The model under review builds one solid part; all positions refer to its coordinate system, in mm. Face numbers are marked on the shaded views. A direction names the side the tool comes from. Round coordinates to 2 decimals unless told otherwise and drop trailing zeros. Write each loop counter-clockwise with the first axis right and the second up, starting at its lowest first coordinate (ties: lowest second). Pieces come first, ordered by that corner, then holes. Notation, with made-up numbers: (64, -36.5) -> (122, -36.5) arc R28 cw to (122, -6.5) -> close; hole circle Ø11 at (30.5, 1). An arc over 180 degrees is marked (long way). Use CSV: the item, a comma, the result in double quotes. Start each with the question number.
1) Machinability: for the marked faces 1 and 2, which of the approach directions +Z, -Z, +X, -X, +Y, -Y give a long, thin tool a straight path to every point of the face, cutting with its end or side? Answer none if there is none.
2) Wall thickness on probe 1 along Y at (x, z) = (0, 1.2); probe 2 along X at (y, z) = (3, 4); probe 3 along Y at (x, z) = (1, 3.6): over which ranges is each line inside the solid? List them lowest first. Write a range as [from, to].
3) Take a section at A-A, the plane y = 0. State how many separate pieces and enclosed holes the cut face has, then the cut area to 3 significant figures.
4) Mouldability with a two-part tool opening along X and no side actions: class the marked faces 3 and 4 as released by +X, released by -X, zero draft, split by the parting line, or undercut.
5) For pin 1 Ø8.5 at (x, y) = (-29, 0) entering from +Z; pin 2 Ø18.5 at (x, y) = (-7, -2) entering from -Z; pin 3 Ø1 at (y, z) = (-20, 1) entering from +X, all flat-tipped, find the tip position at first contact; note any pin that passes through.
6) Take a section at B-B, the plane z = 3.3. Give the boundary of the cut face in (x, y).
from build123d import *

# Parameters (mm, degrees)
F0_R     = 37
F0_R_2   = 3.25
F1_DEPTH = 5
F2_SIZE  = 2.75
F3_SIZE  = 0.5
F4_R     = 19
F5_DEPTH = 2
F6_SIZE  = 0.5


with BuildPart() as f1:
    # F0 (on Top) → F1 (new body)
    with BuildSketch(Plane.XY):
        Circle(F0_R)
        with Locations((0, -29)):
            Circle(F0_R_2, mode=Mode.SUBTRACT)
        with Locations((-29, 0)):
            Circle(F0_R_2, mode=Mode.SUBTRACT)
        with Locations((29, 0)):
            Circle(F0_R_2, mode=Mode.SUBTRACT)
        with Locations((0, 29)):
            Circle(F0_R_2, mode=Mode.SUBTRACT)
    extrude(amount=F1_DEPTH)

    # F2
    f2_edges = [f1.edges().sort_by_distance(p)[0] for p in [
        (-3.25, -29, 5),
        (-32.25, 0, 5),
        (-3.25, 29, 5),
        (25.75, 0, 5),
    ]]
    chamfer(f2_edges, length=F2_SIZE)

    # F3
    f3_edges = [f1.edges().sort_by_distance(p)[0] for p in [
        (37, 0, 2.5),
        (-37, 0, 0),
        (-37, 0, 5),
        (-3.25, -29, 0),
        (-32.25, 0, 0),
        (-3.25, 29, 0),
        (25.75, 0, 0),
    ]]
    chamfer(f3_edges, length=F3_SIZE)

    # F4 (on face) → F5 (cut)
    with BuildSketch(Plane(origin=(0, 0, 0), x_dir=(1, 0, 0), z_dir=(0, 0, -1))):
        Circle(F4_R)
    extrude(amount=-F5_DEPTH, mode=Mode.SUBTRACT)

    # F6
    f6_edges = [f1.edges().sort_by_distance(p)[0] for p in [
        (19, 0, 1),
        (-19, 0, 0),
        (-19, 0, 2),
    ]]
    chamfer(f6_edges, length=F6_SIZE)


solid = f1.part
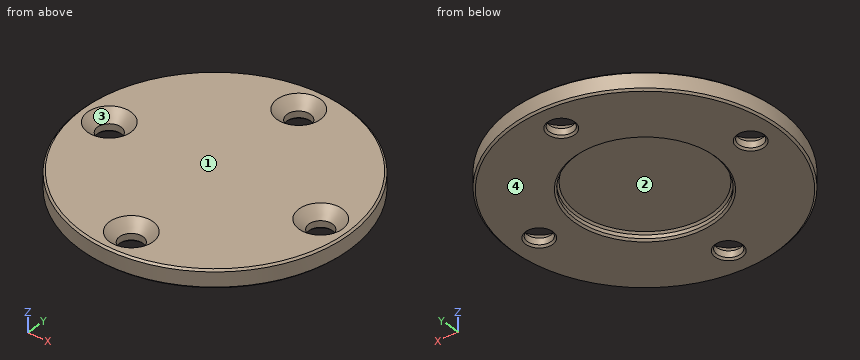
Values found:
1,face 1,"+Z, +X, -X, +Y, -Y"
1,face 2,"-Z"
2,probe 1,"[-37, -32.25], [-25.75, -19], [19, 25.75], [32.25, 37]"
2,probe 2,"[-36.88, -33], [-25, 25], [33, 36.88]"
2,probe 3,"[-36.99, -33.49], [-24.51, 24.51], [33.49, 36.99]"
3,separate pieces,"3"
3,enclosed holes,"0"
3,area,"213 mm²"
4,face 3,"undercut"
4,face 4,"zero draft"
5,pin 1,"z = 3.25"
5,pin 2,"z = 2"
5,pin 3,"x = 31.44"
6,outline,"circle Ø74 at (0, 0); hole circle Ø8.6 at (-29, 0); hole circle Ø8.6 at (0, -29); hole circle Ø8.6 at (0, 29); hole circle Ø8.6 at (29, 0)"
